Read the model definition and answer for the solid it produces. Units are mm, in the model's axes. Give positions to 0.01 mm unless a question says otherwise; leave off trailing zeros. Order: outer loops, then holes, each group sorted by start corner. A loop starts at its lowest first (then second) coordinate and runs counter-clockwise, first axis right, second up. Notation, with made-up numbers: (21.5, 28) - (29.5, 28) arc R9 ccw to (29.5, 39) - close; hole circle Ø3 at (4.25, 35). An arc over 180 degrees is marked (long way). One line per item, written item: value. Start each with the question number.
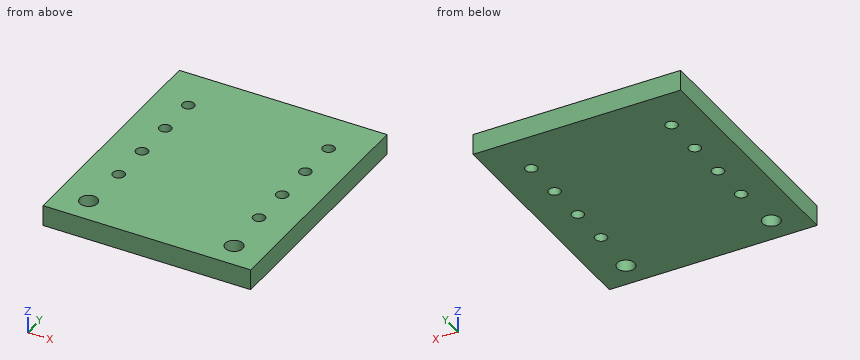
Solid Edge part; units mm, degrees
sketch "Sketch1" plane through (0, 0, 0) normal (0, 0, 1) x (1, 0, 0)
  line L0 (-20, -8) -> (20, -8)
  line L1 (20, -8) -> (20, 39)
  line L2 (20, 39) -> (-20, 39)
  line L3 (-20, 39) -> (-20, -8)
  circle A0 centre (-13.5, 6.5) radius 1.15
  circle A1 centre (-13.5, 14.5) radius 1.15
  circle A2 centre (-13.5, 22.5) radius 1.15
  circle A3 centre (-13.5, 30.5) radius 1.15
  circle A4 centre (13.5, 6.5) radius 1.15
  circle A5 centre (13.5, 14.5) radius 1.15
  circle A6 centre (13.5, 22.5) radius 1.15
  circle A7 centre (13.5, 30.5) radius 1.15
  circle A8 centre (-14, -3) radius 1.7
  circle A9 centre (14, -3) radius 1.7
extrude "Protrusion1" add sketch "Sketch1" along normal blind 4
1) Section A-A on y = 30.5 is taken. Write down the section's boundary in (x, z).
2) Section C-C on x = 13.5 is taken. Write down the section's boundary in (y, z), plus the area to 3 significant figures.
3) Find the intervals of material crossed by probe 1 along Y at (x, z) = (13.5, 2.1); probe 2 along Y at (x, z) = (14, 2.8); probe 3 along X at (y, z) = (31.5, 1.4), in increasing order. Write a range as from..to.
4) Section D-D on y = -3 is taken. Write down the section's boundary in (x, z).
5) Section B-B on z = 0.6 is taken. Give the number of separate pieces and of enclosed holes in the cut face, plus the area to 3 significant figures.
Solved:
1. outline: (-20, 0) - (-14.65, 0) - (-14.65, 4) - (-20, 4) - close; (-12.35, 0) - (12.35, 0) - (12.35, 4) - (-12.35, 4) - close; (14.65, 0) - (20, 0) - (20, 4) - (14.65, 4) - close
2. outline: (-8, 0) - (-4.62, 0) - (-4.62, 4) - (-8, 4) - close; (-1.38, 0) - (5.35, 0) - (5.35, 4) - (-1.38, 4) - close; (7.65, 0) - (13.35, 0) - (13.35, 4) - (7.65, 4) - close; (15.65, 0) - (21.35, 0) - (21.35, 4) - (15.65, 4) - close; (23.65, 0) - (29.35, 0) - (29.35, 4) - (23.65, 4) - close; (31.65, 0) - (39, 0) - (39, 4) - (31.65, 4) - close
2. area: 138 mm2
3. probe 1: y = -8..-4.62, -1.38..5.35, 7.65..13.35, 15.65..21.35, 23.65..29.35, 31.65..39
3. probe 2: y = -8..-4.7, -1.3..5.46, 7.54..13.46, 15.54..21.46, 23.54..29.46, 31.54..39
3. probe 3: x = -20..-14.07, -12.93..12.93, 14.07..20
4. outline: (-20, 0) - (-15.7, 0) - (-15.7, 4) - (-20, 4) - close; (-12.3, 0) - (12.3, 0) - (12.3, 4) - (-12.3, 4) - close; (15.7, 0) - (20, 0) - (20, 4) - (15.7, 4) - close
5. separate pieces: 1
5. enclosed holes: 10
5. area: 1,830 mm2
